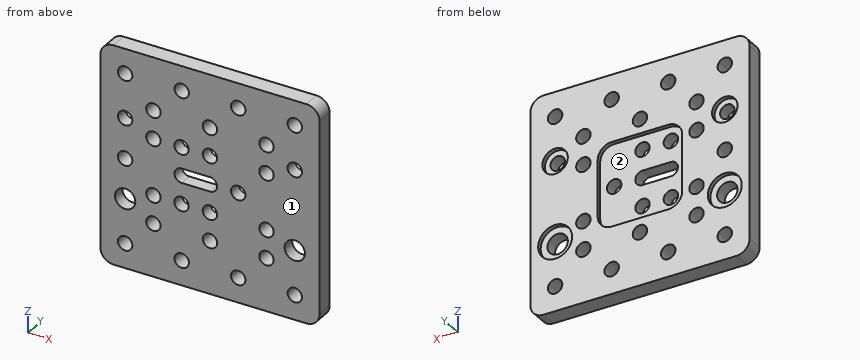
```python
from build123d import *

# Parameters (mm, degrees)
SKETCH1_R           = 2.55
SKETCH1_R_2         = 3.6
BOSS_EXTRUDE1_DEPTH = 6
SKETCH2_R           = 6
SKETCH2_R_2         = 4.5
CUT_EXTRUDE1_DEPTH  = 1.5


with BuildPart() as part:
    # Sketch1 → Boss-Extrude1 (new body)
    with BuildSketch(Plane(origin=(0, 0, 0), x_dir=(1, 0, 0), z_dir=(0, 1, 0))):
        with BuildLine():
            Line((-34.12, 0), (34.12, 0))
            ThreePointArc((34.12, 0), (37.397439931, 1.357560069), (38.755, 4.635))
            Line((38.755, 4.635), (38.755, 72.884))
            ThreePointArc((38.755, 72.884), (37.397439931, 76.161439931), (34.12, 77.519))
            Line((34.12, 77.519), (-34.12, 77.519))
            ThreePointArc((-34.12, 77.519), (-37.397439931, 76.161439931), (-38.755, 72.884))
            Line((-38.755, 72.884), (-38.755, 4.635))
            ThreePointArc((-38.755, 4.635), (-37.397439931, 1.357560069), (-34.12, 0))
        make_face()
        with Locations((-10, 68.76)):
            Circle(SKETCH1_R, mode=Mode.SUBTRACT)
        with Locations((-30, 68.76)):
            Circle(SKETCH1_R, mode=Mode.SUBTRACT)
        with Locations((10, 68.76)):
            Circle(SKETCH1_R, mode=Mode.SUBTRACT)
        with Locations((30, 68.76)):
            Circle(SKETCH1_R, mode=Mode.SUBTRACT)
        with Locations((-30, 8.759)):
            Circle(SKETCH1_R, mode=Mode.SUBTRACT)
        with Locations((-10, 8.759)):
            Circle(SKETCH1_R, mode=Mode.SUBTRACT)
        with Locations((10, 8.759)):
            Circle(SKETCH1_R, mode=Mode.SUBTRACT)
        with Locations((30, 8.759)):
            Circle(SKETCH1_R, mode=Mode.SUBTRACT)
        with Locations((0, 58.76)):
            Circle(SKETCH1_R, mode=Mode.SUBTRACT)
        with Locations((-20, 58.76)):
            Circle(SKETCH1_R, mode=Mode.SUBTRACT)
        with Locations((20, 58.76)):
            Circle(SKETCH1_R, mode=Mode.SUBTRACT)
        with Locations((20, 18.759)):
            Circle(SKETCH1_R, mode=Mode.SUBTRACT)
        with Locations((0, 18.759)):
            Circle(SKETCH1_R, mode=Mode.SUBTRACT)
        with Locations((-20, 18.759)):
            Circle(SKETCH1_R, mode=Mode.SUBTRACT)
        with Locations((-20, 48.7595)):
            Circle(SKETCH1_R, mode=Mode.SUBTRACT)
        with Locations((0, 48.7595)):
            Circle(SKETCH1_R, mode=Mode.SUBTRACT)
        with Locations((20, 48.7595)):
            Circle(SKETCH1_R, mode=Mode.SUBTRACT)
        with Locations((-10.05, 48.7595)):
            Circle(SKETCH1_R, mode=Mode.SUBTRACT)
        with Locations((20, 28.7595)):
            Circle(SKETCH1_R, mode=Mode.SUBTRACT)
        with Locations((0, 28.7595)):
            Circle(SKETCH1_R, mode=Mode.SUBTRACT)
        with Locations((-10.05, 28.7595)):
            Circle(SKETCH1_R, mode=Mode.SUBTRACT)
        with Locations((-20, 28.7595)):
            Circle(SKETCH1_R, mode=Mode.SUBTRACT)
        with Locations((10, 38.7595)):
            Circle(SKETCH1_R, mode=Mode.SUBTRACT)
        with Locations((-30, 38.7595)):
            Circle(SKETCH1_R, mode=Mode.SUBTRACT)
        with Locations((-30, 53.01)):
            Circle(SKETCH1_R_2, mode=Mode.SUBTRACT)
        with Locations((-30, 24.509)):
            Circle(SKETCH1_R, mode=Mode.SUBTRACT)
        with Locations((30, 24.509)):
            Circle(SKETCH1_R, mode=Mode.SUBTRACT)
        with Locations((30, 53.01)):
            Circle(SKETCH1_R_2, mode=Mode.SUBTRACT)
        with BuildLine():
            Line((0, 36.2095), (-10, 36.2095))
            ThreePointArc((-10, 36.2095), (-12.55, 38.7595), (-10, 41.3095))
            Line((-10, 41.3095), (0, 41.3095))
            ThreePointArc((0, 41.3095), (2.55, 38.7595), (0, 36.2095))
        make_face(mode=Mode.SUBTRACT)
    extrude(amount=BOSS_EXTRUDE1_DEPTH)

    # Sketch2 → Cut-Extrude1 (cut)
    with BuildSketch(Plane(origin=(0, 6, 0), x_dir=(1, 0, 0), z_dir=(0, 1, 0))):
        with Locations((-30, 53.01)):
            Circle(SKETCH2_R)
        with Locations((-30, 24.509)):
            Circle(SKETCH2_R_2)
        with Locations((30, 53.01)):
            Circle(SKETCH2_R)
        with Locations((30, 24.509)):
            Circle(SKETCH2_R_2)
        with BuildLine():
            Line((-10.03, 53.7095), (10.03, 53.7095))
            ThreePointArc((10.03, 53.7095), (13.50967247, 52.26817247), (14.951, 48.7885))
            Line((14.951, 48.7885), (14.951, 28.7305))
            ThreePointArc((14.951, 28.7305), (13.50967247, 25.25082753), (10.03, 23.8095))
            Line((10.03, 23.8095), (-10.03, 23.8095))
            ThreePointArc((-10.03, 23.8095), (-13.50967247, 25.25082753), (-14.951, 28.7305))
            Line((-14.951, 28.7305), (-14.951, 48.7885))
            ThreePointArc((-14.951, 48.7885), (-13.50967247, 52.26817247), (-10.03, 53.7095))
        make_face()
    extrude(amount=-CUT_EXTRUDE1_DEPTH, mode=Mode.SUBTRACT)


solid = part.part
```
CAD build for the part. Positions are in the model's coordinates, mm. Face numbers are marked on the shaded views. Give positions to 0.01 mm unless a question says otherwise; leave off trailing zeros. Write each loop counter-clockwise with the first axis right and the second up, starting at its lowest first coordinate (ties: lowest second). Pieces come first, ordered by that corner, then holes. Notation, with made-up numbers: (-20.75, -7.5) -> (33.25, -7.5) arc R21 cw to (33.25, 13.5) -> close; hole circle Ø2 at (52.5, -34). An arc over 180 degrees is marked (long way). Write each question's results on one line, items separated by ' | '.
1. Two-plate mould, pull along Z, no slides. Class the marked faces 1 and 2: pulls with the +Z half, pulls with the -Z half, needs draft (parallel to the pull), parting line crosses it, or undercut.
Geometry check:
face 1: needs draft | face 2: undercut
2. Cut at B-B, the plane z = -68.76. Write the cut outline in (x, y) (3 decimals), then the cut area to 3 significant figures.
Geometry check:
outline: (-38.755, 0) -> (-32.55, 0) -> (-32.55, 6) -> (-38.755, 6) -> close; (-27.45, 0) -> (-12.55, 0) -> (-12.55, 6) -> (-27.45, 6) -> close; (-7.45, 0) -> (7.45, 0) -> (7.45, 6) -> (-7.45, 6) -> close; (12.55, 0) -> (27.45, 0) -> (27.45, 6) -> (12.55, 6) -> close; (32.55, 0) -> (38.755, 0) -> (38.755, 6) -> (32.55, 6) -> close | area: 343 mm²
3. Wall check: probe 1 along Z at (x, y) = (10, 3.25); probe 2 along Z at (x, y) = (-30, 3.15); probe 3 along X at (y, z) = (4.15, -29) (3 decimals). Give the ranges that are in metal, low to high. Write a range as [from, to].
Geometry check:
probe 1: [-77.52, -71.31], [-66.21, -41.31], [-36.21, -11.31], [-6.21, 0] | probe 2: [-77.52, -71.31], [-66.21, -56.61], [-49.41, -41.31], [-36.21, -27.06], [-21.96, -11.31], [-6.21, 0] | probe 3: [-38.755, -22.539], [-17.461, -12.589], [-7.511, -2.539], [2.539, 17.461], [22.539, 38.755]
4. Cut at C-C, the plane x = -20. Write the cut outline in (y, z), then the cut area to 3 significant figures.
Geometry check:
outline: (0, -77.52) -> (6, -77.52) -> (6, -61.31) -> (0, -61.31) -> close; (0, -56.21) -> (6, -56.21) -> (6, -51.31) -> (0, -51.31) -> close; (0, -46.21) -> (6, -46.21) -> (6, -31.31) -> (0, -31.31) -> close; (0, -26.21) -> (6, -26.21) -> (6, -21.31) -> (0, -21.31) -> close; (0, -16.21) -> (6, -16.21) -> (6, 0) -> (0, 0) -> close | area: 343 mm²
5. Cut at D-D, the plane x = 9. Write the cut outline in (y, z).
Geometry check:
outline: (0, -77.52) -> (6, -77.52) -> (6, -71.11) -> (0, -71.11) -> close; (0, -66.41) -> (6, -66.41) -> (6, -53.71) -> (4.5, -53.71) -> (4.5, -41.11) -> (0, -41.11) -> close; (0, -36.41) -> (4.5, -36.41) -> (4.5, -23.81) -> (6, -23.81) -> (6, -11.1) -> (0, -11.1) -> close; (0, -6.41) -> (6, -6.41) -> (6, 0) -> (0, 0) -> close
6. Drop a flat-ended pin along its axis: P1, Ø9, axis at x = 0.5, z = -45, coming from the +Y side. Give the stop position or say it passes through.
Geometry check:
P1: y = 4.5
7. Cut at A-A, the plane x = -30. Give the number of separate pieces and of enclosed holes in the cut face, then the cut area to 3 significant figures.
Geometry check:
separate pieces: 6 | enclosed holes: 0 | area: 286 mm²
